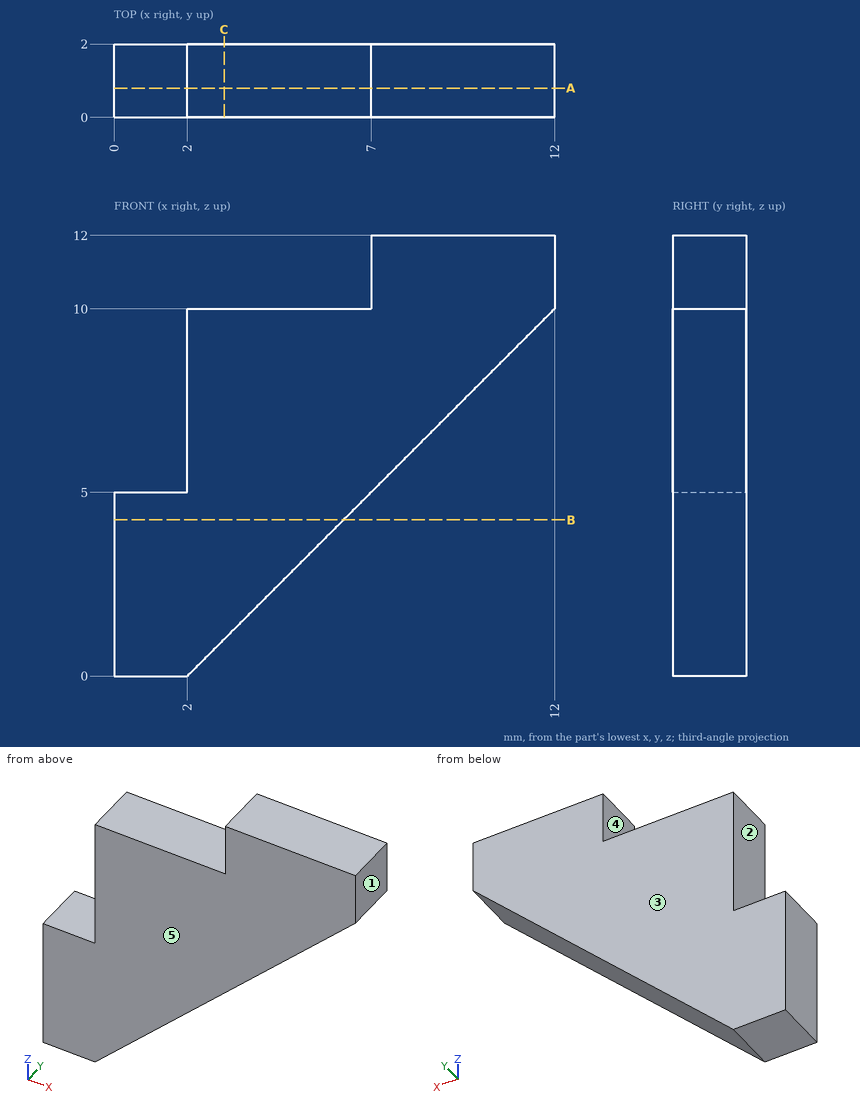
Geometry: see drawing. Coordinates: mm, zero at the bounding-box minimum. A direction names the side the tool comes from. Coordinates: 2 decimals unless noted, no trailing zeros. Write each loop counter-clockwise with the first axis right and the second up, starting at its lowest first coordinate (ties: lowest second). Pieces come first, ordered by that corner, then holes.
1) Mould query, pull axis Y, two halves, no side actions, for the marked faces 3, 4 and 5. Classes: pulls with the +Y half, pulls with the -Y half, needs draft (parallel to the pull), parting line crosses it, or undercut.
2) Pin query (flat end, axial travel): pin 1 Ø0.6 at (y, z) = (1.5, 11) entering from -X. Return the tip coordinate at first contact, or that it passes through.
3) Section B-B on z = 4.25. Output: boundary loops of the cut face in (x, y).
4) Material intervals for line 1 along Z through (x, y) = (9, 1.55); line 2 along Z through (x, y) = (8.75, 1), sorted ascending.
5) Set-up query: the marked faces 1 and 2. Return all of +Z, -Z, +X, -X, +Y, -Y with unobstructed straight access to the full face (end or side cutting, diameter ignored); none if empty.
6) Section C-C on x = 3. Output: boundary loops of the cut face in (y, z), and give its area (3 significant figures).
7) Section A-A on y = 0.8. Output: boundary loops of the cut face in (x, z), and give its area (3 significant figures).
Check result:
1. face 3: pulls with the +Y half
1. face 4: needs draft
1. face 5: pulls with the -Y half
2. pin 1: stops at x = 7
3. outline: (0, 0) - (6.25, 0) - (6.25, 2) - (0, 2) - close
4. line 1: z = 7 to 12
4. line 2: z = 6.75 to 12
5. face 1: +Z, -Z, +X, +Y, -Y
5. face 2: +Z, -X, +Y, -Y
6. outline: (0, 1) - (2, 1) - (2, 10) - (0, 10) - close
6. area: 18.0 mm2
7. outline: (0, 0) - (2, 0) - (12, 10) - (12, 12) - (7, 12) - (7, 10) - (2, 10) - (2, 5) - (0, 5) - close
7. area: 70.0 mm2
